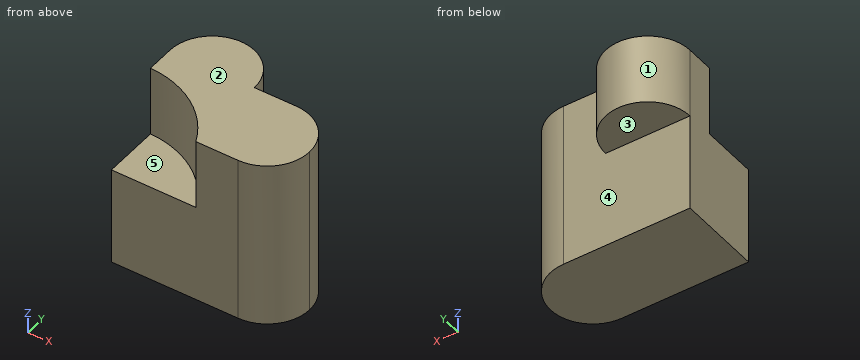
from build123d import *

# Parameters (mm, degrees)
SKETCH1_W               = 6
SKETCH1_H               = 6
BOSS_EXTRUDE1_DEPTH     = 5
CUT_EXTRUDE1_DEPTH      = 10
CUT_EXTRUDE2_DEPTH      = 1
CUT_EXTRUDE2_DEPTH_BACK = 2.5
SKETCH4_W               = 3.5
SKETCH4_H               = 1.5
CUT_EXTRUDE3_DEPTH      = 12.5


with BuildPart() as part:
    # Sketch1 → Boss-Extrude1 (new body)
    with BuildSketch(Plane(origin=(0, 0, 0), x_dir=(1, 0, 0), z_dir=(0, 1, 0))):
        Rectangle(SKETCH1_W, SKETCH1_H)
    extrude(amount=BOSS_EXTRUDE1_DEPTH)

    # Sketch2 → Cut-Extrude1 (cut)
    with BuildSketch(Plane.XY.offset(3)):
        with BuildLine():
            ThreePointArc((-3, 3), (-1.5, 4.5), (0, 3))
            Line((0, 3), (1.5, 3))
            ThreePointArc((1.5, 3), (2.560660172, 2.560660172), (3, 1.5))
            Line((3, 1.5), (3, 5))
            Line((3, 5), (-3, 5))
            Line((-3, 5), (-3, 3))
        make_face()
        with BuildLine():
            Line((3, 0), (3, 1.5))
            ThreePointArc((3, 1.5), (2.560660172, 0.439339828), (1.5, 0))
            Line((1.5, 0), (3, 0))
        make_face()
    extrude(amount=-CUT_EXTRUDE1_DEPTH, mode=Mode.SUBTRACT)

    # Sketch3 → Cut-Extrude2 (cut, two sides)
    with BuildSketch(Plane.XY.offset(3)) as cut_extrude2_sk:
        with BuildLine():
            Line((-3, 2), (-3, 0))
            Line((-3, 0), (0, 0))
            ThreePointArc((0, 0), (-1.210432595, 1.434351108), (-3, 2))
        make_face()
    extrude(amount=CUT_EXTRUDE2_DEPTH, mode=Mode.SUBTRACT)
    extrude(cut_extrude2_sk.sketch, amount=-CUT_EXTRUDE2_DEPTH_BACK, mode=Mode.SUBTRACT)

    # Sketch4 → Cut-Extrude3 (cut)
    with BuildSketch(Plane.ZY.offset(3)):
        with Locations((-1.25, 3.75)):
            Rectangle(SKETCH4_W, SKETCH4_H)
    extrude(amount=-CUT_EXTRUDE3_DEPTH, mode=Mode.SUBTRACT)


solid = part.part
Build history of the part. All positions in model axes, mm. Face numbers are marked on the shaded views. A direction names the side the tool comes from. Coordinates: 2 decimals unless noted, no trailing zeros. Write each loop counter-clockwise with the first axis right and the second up, starting at its lowest first coordinate (ties: lowest second). Pieces come first, ordered by that corner, then holes. Notation, with made-up numbers: (54.5, 44) -> (109.5, 44) arc R21 cw to (109.5, 63) -> close; hole circle Ø3 at (-31.5, 60). An arc over 180 degrees is marked (long way). Use CSV: the item, a comma, the result in double quotes. Start each with the question number.
Q1. Cut at B-B, the plane x = -0.2. List the corners of the cut face in (y, z).
Q2. Cut at A-A, the plane z = 1.3. List the corners of the cut face in (x, y), then the cut area to 3 significant figures.
Q3. Cut at D-D, the plane z = 0.15. List the corners of the cut face in (x, y).
Q4. 3-axis set-ups, long thin cutter, end or side, ignore diameter. For the marked faces 1, 2, 3, 4 and 5: which of +Z, -Z, +X, -X, +Y, -Y reach the whole face in a straight line?
Q5. Flat gauge pin, fed straight in: pin 1 Ø3.5 at (x, z) = (0, 0) entering from +Y. Where does the tip first touch, or does it go through?
Q6. Cut at C-C, the plane y = 2.4. List the corners of the cut face in (x, z).
Q7. Drill centre lines: probe 1 along Z at (x, y) = (-1.85, 1.05); probe 2 along Y at (x, z) = (-1, -2.5); probe 3 along Y at (x, z) = (1.9, 1.85). Where is each one in solid material? Low to high.
Checked values:
1,outline,"(0, -3) -> (3, -3) -> (3, 0.5) -> (3.75, 0.5) -> (3.75, 3) -> (0.38, 3) -> (0.38, 0.5) -> (0, 0.5) -> close"
2,outline,"(-3, 2) arc R3.37 cw to (0, 0) -> (1.5, 0) arc R1.5 ccw to (1.5, 3) -> (0, 3) arc R1.5 ccw to (-3, 3) -> close"
2,area,"16.3 mm²"
3,outline,"(-3, 0) -> (1.5, 0) arc R1.5 ccw to (1.5, 3) -> (-3, 3) -> close"
4,face 1,"+Z, -Z, +Y"
4,face 2,"+Z, +X, -X, +Y, -Y"
4,face 3,"-Z, +X, -X, +Y"
4,face 4,"-Z, +X, +Y"
4,face 5,"+Z, -X, -Y"
5,pin 1,"stops at y = 4.5"
6,outline,"(-3, -3) -> (2.7, -3) -> (2.7, 3) -> (-3, 3) -> close"
7,probe 1,"z = -3 to 0.5"
7,probe 2,"y = 0 to 3"
7,probe 3,"y = 0.05 to 2.95"
